from build123d import *

# Parameters (mm, degrees)
SKETCH1_R           = 2.5
BOSS_EXTRUDE1_DEPTH = 250


with BuildPart() as part:
    # Sketch1 → Boss-Extrude1 (new body)
    with BuildSketch(Plane(origin=(0, 0, 0), x_dir=(0, 0, -1), z_dir=(1, 0, 0))):
        with BuildLine():
            Line((-10, 10), (-10, 5.3))
            Line((-10, 5.3), (-7.8, 3.1))
            Line((-7.8, 3.1), (-7.8, 5.320101013))
            ThreePointArc((-7.8, 5.320101013), (-7.491341716, 5.782040779), (-6.946446609, 5.673654403))
            Line((-6.946446609, 5.673654403), (-4.585786438, 3.312994231))
            ThreePointArc((-4.585786438, 3.312994231), (-4.152240935, 2.664147534), (-4, 1.898780669))
            Line((-4, 1.898780669), (-4, 0))
            Line((-4, 0), (-4, -1.898780669))
            ThreePointArc((-4, -1.898780669), (-4.152240935, -2.664147534), (-4.585786438, -3.312994231))
            Line((-4.585786438, -3.312994231), (-6.946446609, -5.673654403))
            ThreePointArc((-6.946446609, -5.673654403), (-7.491341716, -5.782040779), (-7.8, -5.320101013))
            Line((-7.8, -5.320101013), (-7.8, -3.1))
            Line((-7.8, -3.1), (-10, -5.3))
            Line((-10, -5.3), (-10, -14.7))
            Line((-10, -14.7), (-7.8, -16.9))
            Line((-7.8, -16.9), (-7.8, -14.679898987))
            ThreePointArc((-7.8, -14.679898987), (-7.491341716, -14.217959221), (-6.946446609, -14.326345597))
            Line((-6.946446609, -14.326345597), (-4.585786438, -16.687005769))
            ThreePointArc((-4.585786438, -16.687005769), (-4.152240935, -17.335852466), (-4, -18.101219331))
            Line((-4, -18.101219331), (-4, -20))
            Line((-4, -20), (-4, -21.898780669))
            ThreePointArc((-4, -21.898780669), (-4.152240935, -22.664147534), (-4.585786438, -23.312994231))
            Line((-4.585786438, -23.312994231), (-6.946446609, -25.673654403))
            ThreePointArc((-6.946446609, -25.673654403), (-7.491341716, -25.782040779), (-7.8, -25.320101013))
            Line((-7.8, -25.320101013), (-7.8, -23.1))
            Line((-7.8, -23.1), (-10, -25.3))
            Line((-10, -25.3), (-10, -30))
            Line((-10, -30), (-5.3, -30))
            Line((-5.3, -30), (-3.1, -27.8))
            Line((-3.1, -27.8), (-5.320101013, -27.8))
            ThreePointArc((-5.320101013, -27.8), (-5.782040779, -27.491341716), (-5.673654403, -26.946446609))
            Line((-5.673654403, -26.946446609), (-3.312994231, -24.585786438))
            ThreePointArc((-3.312994231, -24.585786438), (-2.664147534, -24.152240935), (-1.898780669, -24))
            Line((-1.898780669, -24), (1.898780669, -24))
            ThreePointArc((1.898780669, -24), (2.664147534, -24.152240935), (3.312994231, -24.585786438))
            Line((3.312994231, -24.585786438), (5.673654403, -26.946446609))
            ThreePointArc((5.673654403, -26.946446609), (5.782040779, -27.491341716), (5.320101013, -27.8))
            Line((5.320101013, -27.8), (3.1, -27.8))
            Line((3.1, -27.8), (5.3, -30))
            Line((5.3, -30), (10, -30))
            Line((10, -30), (10, -25.3))
            Line((10, -25.3), (7.8, -23.1))
            Line((7.8, -23.1), (7.8, -25.320101013))
            ThreePointArc((7.8, -25.320101013), (7.491341716, -25.782040779), (6.946446609, -25.673654403))
            Line((6.946446609, -25.673654403), (4.585786438, -23.312994231))
            ThreePointArc((4.585786438, -23.312994231), (4.152240935, -22.664147534), (4, -21.898780669))
            Line((4, -21.898780669), (4, -20))
            Line((4, -20), (4, -18.101219331))
            ThreePointArc((4, -18.101219331), (4.152240935, -17.335852466), (4.585786438, -16.687005769))
            Line((4.585786438, -16.687005769), (6.946446609, -14.326345597))
            ThreePointArc((6.946446609, -14.326345597), (7.491341716, -14.217959221), (7.8, -14.679898987))
            Line((7.8, -14.679898987), (7.8, -16.9))
            Line((7.8, -16.9), (10, -14.7))
            Line((10, -14.7), (10, -5.3))
            Line((10, -5.3), (7.8, -3.1))
            Line((7.8, -3.1), (7.8, -5.320101013))
            ThreePointArc((7.8, -5.320101013), (7.491341716, -5.782040779), (6.946446609, -5.673654403))
            Line((6.946446609, -5.673654403), (4.585786438, -3.312994231))
            ThreePointArc((4.585786438, -3.312994231), (4.152240935, -2.664147534), (4, -1.898780669))
            Line((4, -1.898780669), (4, 0))
            Line((4, 0), (4, 1.898780669))
            ThreePointArc((4, 1.898780669), (4.152240935, 2.664147534), (4.585786438, 3.312994231))
            Line((4.585786438, 3.312994231), (6.946446609, 5.673654403))
            ThreePointArc((6.946446609, 5.673654403), (7.491341716, 5.782040779), (7.8, 5.320101013))
            Line((7.8, 5.320101013), (7.8, 3.1))
            Line((7.8, 3.1), (10, 5.3))
            Line((10, 5.3), (10, 10))
            Line((10, 10), (5.3, 10))
            Line((5.3, 10), (3.1, 7.8))
            Line((3.1, 7.8), (5.320101013, 7.8))
            ThreePointArc((5.320101013, 7.8), (5.782040779, 7.491341716), (5.673654403, 6.946446609))
            Line((5.673654403, 6.946446609), (3.312994231, 4.585786438))
            ThreePointArc((3.312994231, 4.585786438), (2.664147534, 4.152240935), (1.898780669, 4))
            Line((1.898780669, 4), (-1.898780669, 4))
            ThreePointArc((-1.898780669, 4), (-2.664147534, 4.152240935), (-3.312994231, 4.585786438))
            Line((-3.312994231, 4.585786438), (-5.673654403, 6.946446609))
            ThreePointArc((-5.673654403, 6.946446609), (-5.782040779, 7.491341716), (-5.320101013, 7.8))
            Line((-5.320101013, 7.8), (-3.1, 7.8))
            Line((-3.1, 7.8), (-5.3, 10))
            Line((-5.3, 10), (-10, 10))
        make_face()
        Circle(SKETCH1_R, mode=Mode.SUBTRACT)
        with Locations(Location((0, -20, 0), (0, 0, 180))):
            Circle(SKETCH1_R, mode=Mode.SUBTRACT)
        with BuildLine():
            Line((-5.673654403, -6.946446609), (-3.312994231, -4.585786438))
            ThreePointArc((-3.312994231, -4.585786438), (-2.664147534, -4.152240935), (-1.898780669, -4))
            Line((-1.898780669, -4), (1.898780669, -4))
            ThreePointArc((1.898780669, -4), (2.664147534, -4.152240935), (3.312994231, -4.585786438))
            Line((3.312994231, -4.585786438), (5.673654403, -6.946446609))
            ThreePointArc((5.673654403, -6.946446609), (6.257616431, -7.336637562), (6.946446609, -7.473654403))
            Line((6.946446609, -7.473654403), (7.3, -7.473654403))
            ThreePointArc((7.3, -7.473654403), (7.653553391, -7.620101013), (7.8, -7.973654403))
            Line((7.8, -7.973654403), (7.8, -12.026345597))
            ThreePointArc((7.8, -12.026345597), (7.653553391, -12.379898987), (7.3, -12.526345597))
            Line((7.3, -12.526345597), (6.946446609, -12.526345597))
            ThreePointArc((6.946446609, -12.526345597), (6.257616431, -12.663362438), (5.673654403, -13.053553391))
            Line((5.673654403, -13.053553391), (3.312994231, -15.414213562))
            ThreePointArc((3.312994231, -15.414213562), (2.664147534, -15.847759065), (1.898780669, -16))
            Line((1.898780669, -16), (-1.898780669, -16))
            ThreePointArc((-1.898780669, -16), (-2.664147534, -15.847759065), (-3.312994231, -15.414213562))
            Line((-3.312994231, -15.414213562), (-5.673654403, -13.053553391))
            ThreePointArc((-5.673654403, -13.053553391), (-6.257616431, -12.663362438), (-6.946446609, -12.526345597))
            Line((-6.946446609, -12.526345597), (-7.3, -12.526345597))
            ThreePointArc((-7.3, -12.526345597), (-7.653553391, -12.379898987), (-7.8, -12.026345597))
            Line((-7.8, -12.026345597), (-7.8, -7.973654403))
            ThreePointArc((-7.8, -7.973654403), (-7.653553391, -7.620101013), (-7.3, -7.473654403))
            Line((-7.3, -7.473654403), (-6.946446609, -7.473654403))
            ThreePointArc((-6.946446609, -7.473654403), (-6.257616431, -7.336637562), (-5.673654403, -6.946446609))
        make_face(mode=Mode.SUBTRACT)
    extrude(amount=BOSS_EXTRUDE1_DEPTH)


solid = part.part
Can you work these out from the model? Positions are in its coordinate system, mm. A direction names the side the tool comes from. Give positions to 0.01 mm unless a question says otherwise; leave off trailing zeros. Write each question's results on one line, items separated by ' | '.
1) Suppose I cut it at A-A, the plane x = 33.5. Give the number of separate pieces and of enclosed holes in the cut face, then the cut area to 3 significant figures.
Final values:
separate pieces: 1 | enclosed holes: 3 | area: 303 mm^2
2) I'm going to push flat-ended pins straight in: pin 1 Ø1 at (x, z) = (105, 3) entering from -Y; pin 2 Ø3 at (x, z) = (66, 0) entering from -Y; pin 3 Ø0.7 at (x, z) = (84.5, -4.5) entering from +Y; pin 4 Ø6 at (x, z) = (125, 5) entering from +Y. Where does each tip first touch, or does it pass through?
Final values:
pin 1: stops at y = -28.2 | pin 2: stops at y = -24 | pin 3: stops at y = 9.55 | pin 4: stops at y = 10
3) On a 3-axis mill with a long thin cutter (end or side, diameter ignored), from which of +Z, -Z, +X, -X, +Y, -Y can I reach the whole of each face in a straight line? I mean faces 4 (the face through (123, -30, 8)), 5 (the face through (123, -10, -7.8)). Say none if no direction works.
Final values:
face 4: +Z, -Z, +X, -X, -Y | face 5: +X, -X
4) Please list where these lines run through material, in increasing order: line 1 along Y through (x, z) = (94, 0); line 2 along Y through (x, z) = (168, 7); line 3 along Y through (x, z) = (206, 9.25). Write a range as [from, to].
Final values:
line 1: y = [-24, -22.5], [-17.5, -16], [-4, -2.5], [2.5, 4] | line 2: y = [-30, -25.72], [-14.28, -12.53], [-7.47, -5.72], [5.72, 10] | line 3: y = [-30, -24.55], [-15.45, -4.55], [4.55, 10]
5) If we mould it in two halves opening along Y, with no side actions, what happens to faces 1 (the face through (123, -30, -8)), 2 (the face through (123.25, -2.44, 0.54)), 3 (the face through (250, -5, -4))? For each: pulls with the +Y half, pulls with the -Y half, needs draft (parallel to the pull), parting line crosses it, or undercut.
Final values:
face 1: pulls with the -Y half | face 2: undercut | face 3: needs draft
